from build123d import *

# Parameters (mm, degrees)
SKETCH1_W           = 25.4
SKETCH1_H           = 50.8
BOSS_EXTRUDE1_DEPTH = 355.6
SHELL1_T            = -3.175
SKETCH2_R           = 2.38125
CUT_EXTRUDE1_DEPTH  = 358.409680899


with BuildPart() as part:
    # Sketch1 → Boss-Extrude1 (new, symmetric)
    with BuildSketch(Plane(origin=(0, 0, 0), x_dir=(0, 0, -1), z_dir=(1, 0, 0))):
        Rectangle(SKETCH1_W, SKETCH1_H)
    extrude(amount=BOSS_EXTRUDE1_DEPTH, both=True)

    # Shell1
    shell1_openings = [part.faces().sort_by_distance(p)[0] for p in [
        (355.6, 0, 0),
        (-355.6, 0, 0),
    ]]
    offset(amount=SHELL1_T, openings=shell1_openings, kind=Kind.INTERSECTION)

    # Sketch2 → Cut-Extrude1 (cut, through all)
    with BuildSketch(Plane.XY.offset(12.7)):
        with Locations((-342.9, 12.7)):
            Circle(SKETCH2_R)
        with Locations((-342.9, 0)):
            Circle(SKETCH2_R)
        with Locations((-342.9, -12.7)):
            Circle(SKETCH2_R)
        with Locations(Location((342.9, -12.7, 0), (0, 0, 180))):
            Circle(SKETCH2_R)
        with Locations(Location((342.9, 0, 0), (0, 0, 180))):
            Circle(SKETCH2_R)
        with Locations(Location((342.9, 12.7, 0), (0, 0, 180))):
            Circle(SKETCH2_R)
    extrude(amount=-CUT_EXTRUDE1_DEPTH, mode=Mode.SUBTRACT)


solid = part.part
Input: part model. Units: mm. Frame: model coordinates. A direction names the side the tool comes from. Coordinates: 2 decimals unless noted, no trailing zeros. Order: outer loops, then holes, each group sorted by start corner. A loop starts at its lowest first (then second) coordinate and runs counter-clockwise, first axis right, second up.
1. Ray query, line 1 along Y through (x, z) = (342.9, -11.35); line 2 along Y through (x, z) = (-170, 5) (3 decimals); line 3 along Z through (x, y) = (-267.5, 17.5) (3 decimals). Return the intervals inside material, ascending.
Checked values:
line 1: y = -25.4 to -15.08, -10.32 to -2.38, 2.38 to 10.32, 15.08 to 25.4
line 2: y = -25.4 to -22.225, 22.225 to 25.4
line 3: z = -12.7 to -9.525, 9.525 to 12.7
2. Draft query along Y for faces 3 (the flat face through (355.6, -2, 10)), 4 (the flat face through (5, 25.4, 0)), 5 (the flat face through (5, 0, -9.525)), 6 (the flat face through (5, -25.4, 0)). Return one class per face: +Y half, -Y half, draft (parallel to the pull), parting line (faces both ways), or undercut.
Checked values:
face 3: draft
face 4: +Y half
face 5: undercut
face 6: -Y half
3. Cut plane A-A, the plane x = -205.5. Return loops of the section in (y, z) (3 decimals).
Checked values:
outline: (-25.4, -12.7) - (25.4, -12.7) - (25.4, 12.7) - (-25.4, 12.7) - close; hole (-22.225, -9.525) - (22.225, -9.525) - (22.225, 9.525) - (-22.225, 9.525) - close
4. Contact query for a flat-ended pin moving along its axis: P1, Ø7.5, axis at x = 342.9, y = 0, coming from the -Z side. Output: stop coordinate, or through.
Checked values:
P1: stops at z = -12.7
5. Cut plane B-B, the plane z = 1.75. Return loops of the section in (x, y) (3 decimals), plus the area to 3 significant figures.
Checked values:
outline: (-355.6, -25.4) - (355.6, -25.4) - (355.6, -22.225) - (-355.6, -22.225) - close; (-355.6, 22.225) - (355.6, 22.225) - (355.6, 25.4) - (-355.6, 25.4) - close
area: 4,520 mm2
6. Access query for faces 1 (the flat face through (5, 0, 12.7)), 2 (the flat face through (5, 22.225, 0)). Directions: +Z, -Z, +X, -X, +Y, -Y. A direction counts if a zero-diameter tool reaches every point of the face in a straight line with its end or side. Return the directions, or none.
Checked values:
face 1: +Z, +X, -X, +Y, -Y
face 2: +X, -X
